CAD build for the part. Positions are in the model's coordinates, mm. Face numbers are marked on the shaded views. Give positions to 0.01 mm unless a question says otherwise; leave off trailing zeros. Write each loop counter-clockwise with the first axis right and the second up, starting at its lowest first coordinate (ties: lowest second). Pieces come first, ordered by that corner, then holes. Notation, with made-up numbers: (20.5, 80.5) - (58.5, 80.5) arc R20 ccw to (58.5, 100.5) - close; hole circle Ø5 at (85, 5.5). An arc over 180 degrees is marked (long way). Put each result on its own line as item: value. Start each with the question number.
1. Drop flat-ended pins along their axis: pin 1 (1.5 mm diameter, centred on x = -9.5, y = 2.5, fed in from -Z); pin 2 (2 mm diameter, centred on y = 3.5, z = -6, fed in from -X); pin 3 (1 mm diameter, centred on x = -9.5, y = 5.5, fed in from -Z). Give the stop position or say it passes through.
2. Mould opens along Z. For the marked faces 1, 2, 3 and 4 say: +Z half, -Z half, draft (parallel to the pull), parting line (faces both ways), or undercut.
3. Cut at C-C on z = 5.75. List the corners of the cut face in (x, y), and give its area (3 significant figures).
4. Cut at A-A on x = 4.5. List the corners of the cut face in (y, z).
5. Wall check: line 1 (X direction, y = 5, z = 5.75); line 2 (Z direction, x = 3.5, y = 3); line 3 (X direction, y = 3, z = -0.5). Give the ranges that are in metal, low to high.
6. Cut at D-D on z = -8. List the corners of the cut face in (x, y), and give its area (3 significant figures).
7. Cut at B-B on y = 6. List the corners of the cut face in (x, z), and give its area (3 significant figures).
Autodesk Inventor part; units mm, degrees
ref_plane "YZ Plane" through (0, 0, 0) normal (1, 0, 0) x (0, 1, 0)
ref_plane "XZ Plane" through (0, 0, 0) normal (0, 1, 0) x (-1, 0, 0)
ref_plane "XY Plane" through (0, 0, 0) normal (0, 0, 1) x (1, 0, 0)
sketch "Sketch1" plane through (0, 0, 0) normal (0, 1, 0) x (-1, 0, 0)
  circle A0 centre (0, 0) radius 6.35
  line L0 (-0.1298, -7.3312) -> (-6.4139, -3.5532)
  line L1 (-6.4139, -3.5532) -> (-6.2841, 3.778)
  line L2 (-6.2841, 3.778) -> (0.1298, 7.3312)
  line L3 (0.1298, 7.3312) -> (6.4139, 3.5532)
  line L4 (6.4139, 3.5532) -> (6.2841, -3.778)
  line L5 (6.2841, -3.778) -> (-0.1298, -7.3312)
  circle A1 centre (0, 0) radius 12.7
  point P0 (3.0772, -5.5546)
  dimension "d0" = 12.7
  dimension "d1" = 25.4
extrude "Extrusion1" add sketch "Sketch1" along normal blind 6.35
properties part number "4-bar intake spacer"
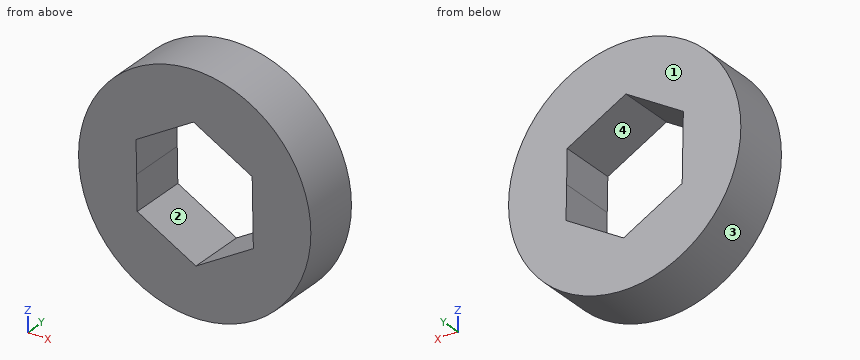
Report:
1. pin 1: stops at z = -9.2
1. pin 2: stops at x = -11.67
1. pin 3: stops at z = -8.96
2. face 1: draft
2. face 2: undercut
2. face 3: parting line
2. face 4: undercut
3. outline: (-11.32, 0) - (-2.76, 0) - (-2.76, 6.35) - (-11.32, 6.35) - close; (2.72, 0) - (11.32, 0) - (11.32, 6.35) - (2.72, 6.35) - close
3. area: 109 mm²
4. outline: (0, -11.88) - (6.35, -11.88) - (6.35, -4.7) - (0, -4.7) - close; (0, 4.77) - (6.35, 4.77) - (6.35, 11.88) - (0, 11.88) - close
5. line 1: x = -11.32 to -2.76, 2.72 to 11.32
5. line 2: z = -12.21 to -5.31, 5.32 to 12.21
5. line 3: x = -12.69 to -6.34, 6.36 to 12.69
6. outline: (-9.86, 0) - (9.86, 0) - (9.86, 6.35) - (-9.86, 6.35) - close
6. area: 125 mm²
7. outline: circle Ø25.4 at (0, 0); hole (-6.41, 3.55) - (-6.28, -3.78) - (0.13, -7.33) - (6.41, -3.55) - (6.28, 3.78) - (-0.13, 7.33) - close
7. area: 367 mm²
